```python
from build123d import *

# Parameters (mm, degrees)
SKETCH1_W           = 50
SKETCH1_H           = 50
SKETCH1_R           = 4
BOSS_EXTRUDE1_DEPTH = 10
FILLET1_R           = 10
FILLET2_R           = 10
SKETCH2_R           = 31.5
BOSS_EXTRUDE2_DEPTH = 50
SKETCH3_R           = 60
SKETCH3_R_2         = 4.15
BOSS_EXTRUDE3_DEPTH = 10
SKETCH4_R           = 17.5
SKETCH4_R_2         = 11
BOSS_EXTRUDE4_DEPTH = 30


with BuildPart() as part:
    # Sketch1 → Boss-Extrude1 (new body)
    # profile 1 of 5: a face of its own
    with BuildSketch(Plane.XY):
        Rectangle(SKETCH1_W, SKETCH1_H)
    # profile 2 of 5: a face of its own
    with BuildSketch(Plane.XY):
        with BuildLine():
            Line((-25, -25), (-25, 25))
            Line((-25, 25), (-33.024481828, 25))
            ThreePointArc((-33.024481828, 25), (-41.42, 0), (-33.024481828, -25))
            Line((-33.024481828, -25), (-25, -25))
        make_face()
        with Locations((-32.935, 0)):
            Circle(SKETCH1_R, mode=Mode.SUBTRACT)
    # profile 3 of 5: a face of its own
    with BuildSketch(Plane.XY):
        with BuildLine():
            Line((25, 25), (25, 33.024481828))
            ThreePointArc((25, 33.024481828), (0, 41.42), (-25, 33.024481828))
            Line((-25, 33.024481828), (-25, 25))
            Line((-25, 25), (25, 25))
        make_face()
        with Locations((0, 32.935)):
            Circle(SKETCH1_R, mode=Mode.SUBTRACT)
    # profile 4 of 5: a face of its own
    with BuildSketch(Plane.XY):
        with BuildLine():
            Line((33.024481828, 25), (25, 25))
            Line((25, 25), (25, -25))
            Line((25, -25), (33.024481828, -25))
            ThreePointArc((33.024481828, -25), (41.42, 0), (33.024481828, 25))
        make_face()
        with Locations((32.935, 0)):
            Circle(SKETCH1_R, mode=Mode.SUBTRACT)
    # profile 5 of 5: a face of its own
    with BuildSketch(Plane.XY):
        with BuildLine():
            Line((25, -33.024481828), (25, -25))
            Line((25, -25), (-25, -25))
            Line((-25, -25), (-25, -33.024481828))
            ThreePointArc((-25, -33.024481828), (0, -41.42), (25, -33.024481828))
        make_face()
        with Locations((0, -32.935)):
            Circle(SKETCH1_R, mode=Mode.SUBTRACT)
    extrude(amount=BOSS_EXTRUDE1_DEPTH)

    # Fillet1
    fillet1_edges = [part.edges().sort_by_distance(p)[0] for p in [
        (-25, 33.024481828, 5),
        (25, 33.024481828, 5),
        (33.024481828, 25, 5),
        (33.024481828, -25, 5),
        (25, -33.024481828, 5),
        (-25, -33.024481828, 5),
        (-33.024481828, -25, 5),
        (-33.024481828, 25, 5),
    ]]
    fillet(fillet1_edges, radius=FILLET1_R)

    # Fillet2
    fillet2_edges = [part.edges().sort_by_distance(p)[0] for p in [
        (25, 25, 5),
        (-25, 25, 5),
        (-25, -25, 5),
        (25, -25, 5),
    ]]
    fillet(fillet2_edges, radius=FILLET2_R)

    # Sketch2 → Boss-Extrude2 (add)
    with BuildSketch(Plane.XY.offset(10)):
        with Locations(Location((0, 0, 0), (0, 0, 173.354533999))):
            Circle(SKETCH2_R)
    extrude(amount=BOSS_EXTRUDE2_DEPTH)

    # Sketch3 → Boss-Extrude3 (add)
    with BuildSketch(Plane.XY.offset(60)):
        Circle(SKETCH3_R)
        with Locations((0, 45)):
            Circle(SKETCH3_R_2, mode=Mode.SUBTRACT)
        with Locations((45, 0)):
            Circle(SKETCH3_R_2, mode=Mode.SUBTRACT)
        with Locations((0, -45)):
            Circle(SKETCH3_R_2, mode=Mode.SUBTRACT)
        with Locations((-45, 0)):
            Circle(SKETCH3_R_2, mode=Mode.SUBTRACT)
    extrude(amount=BOSS_EXTRUDE3_DEPTH)

    # Sketch4 → Boss-Extrude4 (add)
    with BuildSketch(Plane.XY.offset(70)):
        Circle(SKETCH4_R)
        Circle(SKETCH4_R_2, mode=Mode.SUBTRACT)
    extrude(amount=BOSS_EXTRUDE4_DEPTH)


solid = part.part
```
Source: CAD feature listing. Evaluate the final solid. Frame: model axes, mm. A direction names the side the tool comes from. Round coordinates to 2 decimals unless told otherwise and drop trailing zeros. Write each loop counter-clockwise with the first axis right and the second up, starting at its lowest first coordinate (ties: lowest second). Pieces come first, ordered by that corner, then holes. Notation, with made-up numbers: M 35.25,86.25 L 49.25,86.25 A28 cw 49.25,104.25 Z; hole C -19.5,87.25 d1. An arc over 180 degrees is marked long. Answer as a JSON object with one key per item and string values. Group by question number.
(1) Section query A-A on x = 0. State how many separate pieces and enclosed holes the cut face has, then the cut area to 3 significant figures.
(2) Section query D-D on z = 87.5. Output: boundary loops of the cut face in (x, y).
(3) Section query C-C on x = -45. Output: boundary loops of the cut face in (y, z), then the cut area to 3 significant figures.
(4) Mould query, pull axis X, two halves, no side actions, for faces 1 (the cylindrical face through (-22.626, -34.077, 5.07)), 2 (the cylindrical face through (41.42, -0.29, 4.93)), 3 (the cylindrical face through (48.958, 1.247, 64.93)). Classes: +X half, -X half, draft (parallel to the pull), parting line (faces both ways), or undercut.
(5) Reachability of faces 4 (the cylindrical face through (-41.042, 1.247, 64.93)), 5 (the cylindrical face through (0.29, 41.42, 4.93)), 6 (the cylindrical face through (22.69, -34, 5.07)), 7 (the cylindrical face through (27.048, 16.146, 34.65)), 8 (the cylindrical face through (-41.42, 0.29, 4.93)) from +Z, -Z, +X, -X, +Y, -Y: full face, straight path, thin tool, end or side. Return the list, or none.
(6) First-contact query: pin 1 (6.5 mm diameter, centred on x = 0, y = -45, fed in from +Z); pin 2 (4 mm diameter, centred on x = 36, y = -12.5, fed in from +Z); pin 3 (12 mm diameter, centred on x = 4.5, z = 26, fed in from +Y); pin 4 (1 mm diameter, centred on x = 47.5, y = -18.5, fed in from -Z). Flat tips, straight axial feed; report the tip coordinate or a pass-through.
(7) Section query B-B on y = 47.5. Output: boundary loops of the cut face in (x, z).
(8) Ray query, line 1 (Y direction, x = 0, z = 2.5) (3 decimals); line 2 (Y direction, x = 0, z = 68.25); line 3 (Y direction, x = 0, z = 81). Return the intervals inside material, ascending. Write a range as [from, to].
Computed values:
{
 "1": {"separate pieces": "5", "enclosed holes": "0", "area": "5,240 mm^2"},
 "2": {"outline": "C 0,0 d35; hole C 0,0 d22"},
 "3": {"outline": "M -39.69,60 L -4.15,60 L -4.15,70 L -39.69,70 Z; M 4.15,60 L 39.69,60 L 39.69,70 L 4.15,70 Z", "area": "711 mm^2"},
 "4": {"face 1": "-X half", "face 2": "+X half", "face 3": "undercut"},
 "5": {"face 4": "+Z", "face 5": "-Z, +Y", "face 6": "-Z, +X, -Y", "face 7": "none", "face 8": "-Z, -X"},
 "6": {"pin 1": "through", "pin 2": "z = 70", "pin 3": "y = 31.5", "pin 4": "z = 60"},
 "7": {"outline": "M -36.66,60 L -3.31,60 L -3.31,70 L -36.66,70 Z; M 3.31,60 L 36.66,60 L 36.66,70 L 3.31,70 Z"},
 "8": {"line 1": "[-41.42, -36.935], [-28.935, 28.935], [36.935, 41.42]", "line 2": "[-60, -49.15], [-40.85, 40.85], [49.15, 60]", "line 3": "[-17.5, -11], [11, 17.5]"}
}
